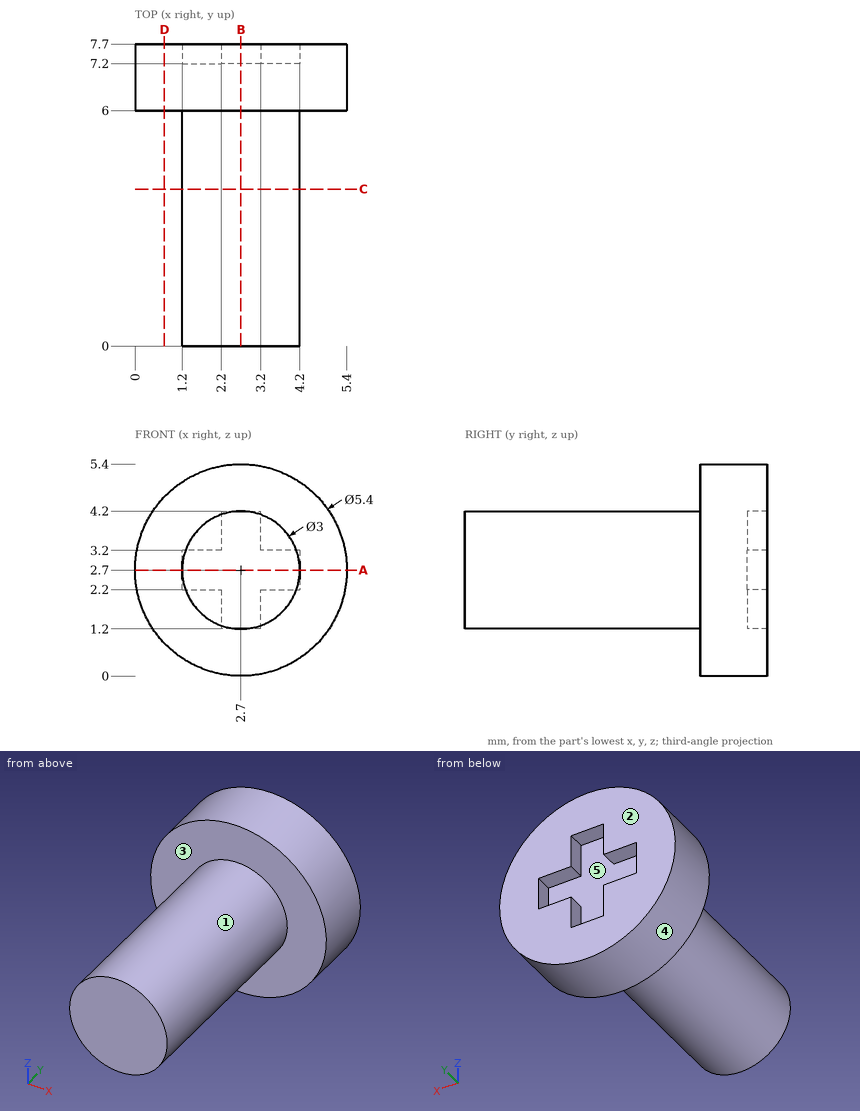
Geometry: see drawing. Coordinates: mm, zero at the bounding-box minimum. A direction names the side the tool comes from. Give positions to 0.01 mm unless a question says otherwise; leave off trailing zeros. Loops run counter-clockwise (first coordinate to the right, second up) from the corner with the lowest first, then second, coordinate; pieces in that order, holes last. Notation, with made-up numbers: (57.5, 67.25) - (82.5, 67.25) arc R22 ccw to (82.5, 84.25) - close; hole circle Ø5 at (31.25, 75). An arc over 180 degrees is marked (long way). Use CSV: the item, a comma, the result in double quotes. Start each with the question number.
Item 1: Section A-A on z = 2.7. Return loops of the section in (x, y).
Item 2: Section D-D on x = 0.75. Return loops of the section in (y, z).
Item 3: Section B-B on x = 2.7. Return loops of the section in (y, z).
Item 4: Line query: line 1 (X direction, y = 4.75, z = 2.7); line 2 (Y direction, x = 1.9, z = 0.6); line 3 (Z direction, x = 2.45, y = 7.25). Output: solid intervals per line, ascending.
Item 5: Reachability of the marked faces 1 and 2 from +Z, -Z, +X, -X, +Y, -Y: full face, straight path, thin tool, end or side. Return the list, or none.
Item 6: Mould query, pull axis X, two halves, no side actions, for the marked faces 3, 4 and 5. Classes: pulls with the +X half, pulls with the -X half, needs draft (parallel to the pull), parting line crosses it, or undercut.
Item 7: Section C-C on y = 4. Return loops of the section in (x, z), then the cut area to 3 significant figures.
Item 8: Contact query for flat-ended pins moving along their axis: P1, Ø2, axis at y = 4.5, z = 3.5, coming from the -X side; P2, Ø0.6, axis at y = 7.5, z = 3.5, coming from the -X side; P3, Ø2, axis at y = 4.5, z = 2, coming from the +X side. Output: stop coordinate, or through.
Ans:
1,outline,"(0, 6) - (1.2, 6) - (1.2, 0) - (4.2, 0) - (4.2, 6) - (5.4, 6) - (5.4, 7.7) - (4.2, 7.7) - (4.2, 7.2) - (1.2, 7.2) - (1.2, 7.7) - (0, 7.7) - close"
2,outline,"(6, 0.83) - (7.7, 0.83) - (7.7, 4.57) - (6, 4.57) - close"
3,outline,"(0, 1.2) - (6, 1.2) - (6, 0) - (7.7, 0) - (7.7, 1.2) - (7.2, 1.2) - (7.2, 4.2) - (7.7, 4.2) - (7.7, 5.4) - (6, 5.4) - (6, 4.2) - (0, 4.2) - close"
4,line 1,"x = 1.2 to 4.2"
4,line 2,"y = 6 to 7.7"
4,line 3,"z = 0.01 to 1.2, 4.2 to 5.39"
5,face 1,"-Y"
5,face 2,"+Z, -Z, +X, -X, +Y"
6,face 3,"needs draft"
6,face 4,"parting line crosses it"
6,face 5,"undercut"
7,outline,"circle Ø3 at (2.7, 2.7)"
7,area,"7.07 mm2"
8,P1,"stops at x = 1.2"
8,P2,"stops at x = 0.05"
8,P3,"stops at x = 4.2"
